Verification items for the finished model (mm, model axes). Give positions to 0.01 mm unless a question says otherwise; leave off trailing zeros. Use one line per item in the form item = value. Start each with the question number.
(1) Section check A-A, the plane z = 0.55. State how many separate pieces and enclosed holes the cut face has, plus the area to 3 significant figures.
(2) Depth check by flat-ended pin: pin 1 Ø4 at (x, y) = (-16, -7.5) entering from -Z. Enter the tip coordinate at first touch or a pass-through.
(3) Scan lines: L1, parallel to X at y = -3.5, z = 1.15; L2, parallel to X at y = -4.5, z = 1.05; L3, parallel to X at y = 19, z = 0.7. Record each from-to range of solid material in increasing order.
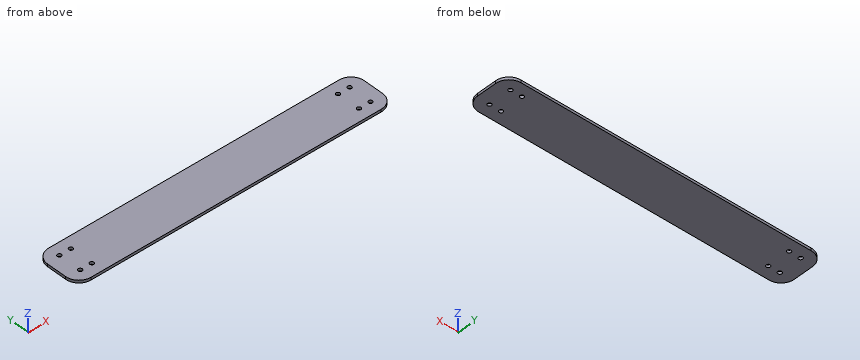
from build123d import *

# Parameters (mm, degrees)
EXTRUDE_1_DEPTH = 2
MM_2_D          = 3
MM_3_D          = 3


with BuildPart() as part:
    # 草图2 → 凸台-拉伸1 (new body)
    with BuildSketch(Plane.XY):
        with BuildLine():
            Line((-50.360367403, 22.370399323), (169.639632597, 22.370399323))
            ThreePointArc((169.639632597, 22.370399323), (176.710700409, 19.441467134), (179.639632597, 12.370399323))
            Line((179.639632597, 12.370399323), (179.639632597, -2.629600677))
            ThreePointArc((179.639632597, -2.629600677), (176.710700409, -9.700668489), (169.639632597, -12.629600677))
            Line((169.639632597, -12.629600677), (-50.360367403, -12.629600677))
            ThreePointArc((-50.360367403, -12.629600677), (-57.431435215, -9.700668489), (-60.360367403, -2.629600677))
            Line((-60.360367403, -2.629600677), (-60.360367403, 12.370399323))
            ThreePointArc((-60.360367403, 12.370399323), (-57.431435215, 19.441467134), (-50.360367403, 22.370399323))
        make_face()
    extrude(amount=EXTRUDE_1_DEPTH)

    # 大小mm 暗销孔2 (through all)
    with Locations(Plane(origin=(-41.610367403, 13.620399323, 0), x_dir=(-1, 0, 0), z_dir=(0, 0, -1))):
        with Locations((0, 0), (8.75, 0), (0, -17.352577314), (8.75, -17.352577314)):
            Hole(MM_2_D / 2)

    # 大小mm 暗销孔3 (through all)
    with Locations(Plane(origin=(169.639632597, 13.620399323, 0), x_dir=(-1, 0, 0), z_dir=(0, 0, -1))):
        with Locations((0, 0), (8.75, 0), (8.75, -17.352577314), (0, -17.352577314)):
            Hole(MM_3_D / 2)


solid = part.part
Completed:
q1.separate_pieces = 1
q1.enclosed_holes = 8
q1.area = 8,260 mm²
q2.pin_1 = 0
q3.L1 = -60.32 to -51.84, -48.88 to -43.09, -40.13 to 159.41, 162.37 to 168.16, 171.12 to 179.6
q3.L2 = -60.18 to -51.65, -49.07 to -42.9, -40.32 to 159.6, 162.18 to 168.35, 170.93 to 179.46
q3.L3 = -57.85 to 177.13
